For this review, take the finished solid that the model builds, in its own axes (mm). Face numbers are marked on the shaded views. Round coordinates to 2 decimals unless told otherwise and drop trailing zeros. Order: outer loops, then holes, each group sorted by start corner. A loop starts at its lowest first (then second) coordinate and runs counter-clockwise, first axis right, second up. Notation, with made-up numbers: M -40,80 L -27,80 A17 ccw -27,103 Z; hole C -2,62.5 d10. An arc over 180 degrees is marked long. Use a Markdown table: item, result.
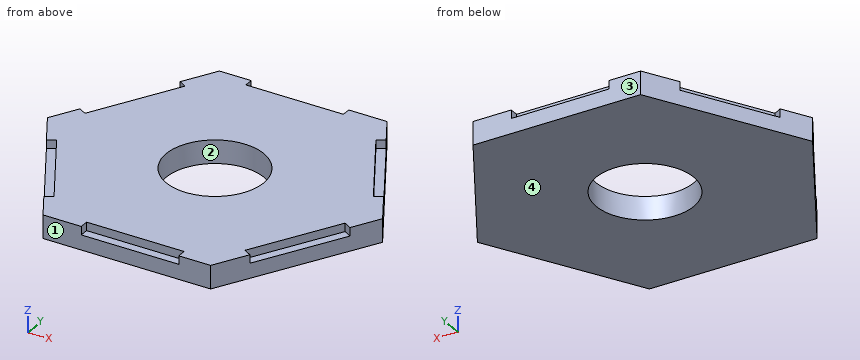
from build123d import *

# Parameters (mm, degrees)
F1_DEPTH        = 6.35
F2_R            = 13.335
F3_DEPTH        = 25.4
F5_DEPTH        = 2.286
F5_COPIES_COUNT = 6


# Not quite as in the source:
# - a pattern or mirror of a feature is missing from the dataset's text; its kind, count and spacing are read off the source's solid


with BuildPart() as f1:
    # F0 (on Top) → F1 (new body)
    with BuildSketch(Plane.XY):
        Polygon((22.9135888085, 39.6875), (-22.9135888085, 39.6875), (-45.8271776169, 0), (-22.9135888085, -39.6875), (22.9135888085, -39.6875), (45.8271776169, 0), align=None)
    extrude(amount=F1_DEPTH)

    # F2 (on face) → F3 (cut)
    with BuildSketch(Plane.XY.offset(6.35)):
        Circle(F2_R)
    extrude(amount=-F3_DEPTH, mode=Mode.SUBTRACT)

    # F4 (on face) → F5 (cut)
    with BuildSketch(Plane.XY.offset(6.35)):
        Polygon((-38.5256609586, -7.8713978245), (-40.5933832127, -9.0651978245), (-27.2583832127, -32.1620953434), (-25.1906609586, -30.9682953434), align=None)
    f5 = extrude(amount=-F5_DEPTH, mode=Mode.SUBTRACT)

    # F5_copies: F5 ×6 about axis
    f5_copies_axis = Axis((0, 0, 0), (0, 0, 1))
    for i in range(1, F5_COPIES_COUNT):
        add(f5.rotate(f5_copies_axis, i * 360 / F5_COPIES_COUNT), mode=Mode.SUBTRACT)


solid = f1.part
Q1. Draft analysis for pull direction Y (two halves, no side actions). For the marked faces 1, 2, 3 and 4, state which applies: pulls with the +Y half, pulls with the -Y half, needs draft (parallel to the pull), parting line crosses it, or undercut.
Determined:
| item | result |
|---|---|
| face 1 | pulls with the -Y half |
| face 2 | undercut |
| face 3 | pulls with the +Y half |
| face 4 | needs draft |
Q2. Clearance check with flat-ended pins moving along their axes: pin 1 (2.5 mm diameter, centred on x = 4.5, y = -39, fed in from +Z); pin 2 (1.1 mm diameter, centred on y = 38, z = 5, fed in from +X); pin 3 (1.8 mm diameter, centred on x = -3, z = 5, fed in from +Y). State where each tip first meets the part, or that it passes through.
Determined:
| item | result |
|---|---|
| pin 1 | stops at z = 4.06 |
| pin 2 | stops at x = 24.21 |
| pin 3 | stops at y = 37.3 |
Q3. Add section D-D (y = 15). Write out the cut boundary in (x, z).
Determined:
| item | result |
|---|---|
| outline | M -37.17,0 L 37.17,0 L 37.17,4.06 L 34.41,4.06 L 34.41,6.35 L -34.41,6.35 L -34.41,4.06 L -37.17,4.06 Z |
Q4. Add section C-C (y = 1.5). Write out the cut boundary in (x, z).
Determined:
| item | result |
|---|---|
| outline | M -44.96,0 L -13.25,0 L -13.25,6.35 L -44.96,6.35 Z; M 13.25,0 L 44.96,0 L 44.96,6.35 L 13.25,6.35 Z |
Q5. Wall thickness on line 1 along Y through (x, z) = (0, 1.75) (1 decimal); line 2 along Y through (x, z) = (-11, 6); line 3 along X through (y, z) = (-4, 0.5): over which ranges is each line inside the solid? List them lowest first. Write a range as [from, to].
Determined:
| item | result |
|---|---|
| line 1 | y = [-39.7, -13.3], [13.3, 39.7] |
| line 2 | y = [-37.3, -7.54], [7.54, 37.3] |
| line 3 | x = [-43.52, -12.72], [12.72, 43.52] |
